Geometry: see drawing. Coordinates: mm, zero at the bounding-box minimum. A direction names the side the tool comes from. Coordinates: 2 decimals unless noted, no trailing zeros. Loops run counter-clockwise (first coordinate to the right, second up) from the corner with the lowest first, then second, coordinate; pieces in that order, holes last. Notation, with made-up numbers: (48.25, -38) -> (81.25, -38) arc R17 ccw to (81.25, -6) -> close; hole circle Ø2 at (28.25, 67.5). An arc over 180 degrees is marked (long way). Put each result on its own line as item: value. Start each with the question number.
1) Contact query for flat-ended pins moving along their axis: P1, Ø2, axis at x = 0.5, y = 0.5, coming from the -Z side; P2, Ø1.5, axis at x = 3.5, y = 3, coming from the +Z side; P3, Ø1, axis at x = 5, y = 2, coming from the +Z side. Output: stop coordinate, or through.
2) Set-up query: the marked faces 1, 2 and 3. Return all of +Z, -Z, +X, -X, +Y, -Y with unobstructed straight access to the full face (end or side cutting, diameter ignored); none if empty.
3) Cut plane B-B (x = 3.1). Return the cut outline in (y, z), plus the area to 3 significant figures.
4) Material intervals for L1, parallel to Y at x = 3.35, z = 2.6; L2, parallel to X at y = 0.45, z = 3.25; L3, parallel to X at y = 3.25, z = 1, sorted ascending.
5) Cut plane A-A (y = 1.15). Return the cut outline in (x, z), plus the area to 3 significant figures.
6) Cut plane D-D (y = 2.15). Return the cut outline in (x, z), plus the area to 3 significant figures.
7) Cut plane C-C (z = 2.3). Return the cut outline in (x, y).
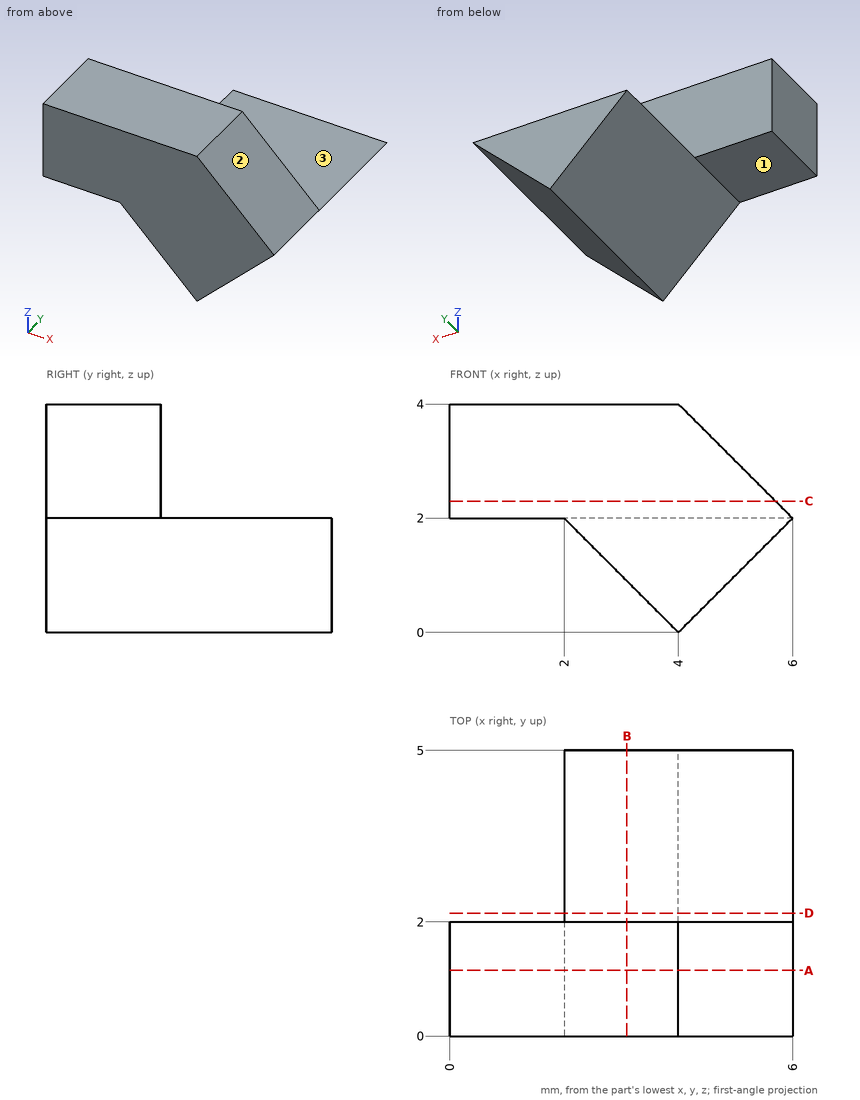
Results found:
1. P1: stops at z = 2
1. P2: stops at z = 2
1. P3: stops at z = 3.5
2. face 1: -Z, -X, +Y, -Y
2. face 2: +Z, +X, +Y, -Y
2. face 3: +Z, +X, -X, +Y
3. outline: (0, 0.9) -> (5, 0.9) -> (5, 2) -> (2, 2) -> (2, 4) -> (0, 4) -> close
3. area: 9.50 mm2
4. L1: y = 0 to 2
4. L2: x = 0 to 4.75
4. L3: x = 3 to 5
5. outline: (0, 2) -> (2, 2) -> (4, 0) -> (6, 2) -> (4, 4) -> (0, 4) -> close
5. area: 14.0 mm2
6. outline: (2, 2) -> (4, 0) -> (6, 2) -> close
6. area: 4.00 mm2
7. outline: (0, 0) -> (5.7, 0) -> (5.7, 2) -> (0, 2) -> close
